```python
from build123d import *

# Parameters (mm, degrees)
SKETCH1_R           = 35
BOSS_EXTRUDE1_DEPTH = 50
SKETCH2_R           = 11.75
CUT_EXTRUDE1_DEPTH  = 21
SKETCH3_R           = 9
CUT_EXTRUDE2_DEPTH  = 5
SKETCH6_R           = 6.35
CUT_EXTRUDE3_DEPTH  = 71.356236397
CUT_EXTRUDE4_START  = -20
SKETCH7_R           = 35
CUT_EXTRUDE4_DEPTH  = 20
SKETCH9_R           = 3.302
CUT_EXTRUDE6_DEPTH  = 58.879184514


with BuildPart() as part:
    # Sketch1 → Boss-Extrude1 (new body)
    with BuildSketch(Plane.XY):
        Circle(SKETCH1_R)
    extrude(amount=BOSS_EXTRUDE1_DEPTH)

    # Sketch2 → Cut-Extrude1 (cut)
    with BuildSketch(Plane.XY.offset(50)):
        with Locations((0, -0.363798412)):
            Circle(SKETCH2_R)
    extrude(amount=-CUT_EXTRUDE1_DEPTH, mode=Mode.SUBTRACT)

    # Sketch3 → Cut-Extrude2 (cut)
    with BuildSketch(Plane.XY.offset(29)):
        Circle(SKETCH3_R)
    extrude(amount=-CUT_EXTRUDE2_DEPTH, mode=Mode.SUBTRACT)

    # Sketch4 → Cut-Revolve1 (revolve, cut)
    with BuildSketch(Plane(origin=(0, 0, 0), x_dir=(0, 0, -1), z_dir=(1, 0, 0))):
        with BuildLine():
            Line((-8.85349547, 5), (-8.85349547, 0))
            Line((-8.85349547, 0), (-29.014540537, 0))
            Line((-29.014540537, 0), (-29.014540537, 8.986487334))
            add(Edge.make_bspline(
                [(-29.014540537, 8.986487334), (-22.084577695, 17.461249934), (-14.611301832, 9.423177176), (-8.85349547, 5)],
                knots=[0, 0, 0, 0, 1, 1, 1, 1], degree=3))
        make_face()
    revolve(axis=Axis((0, 0, 8.85349547), (0, 0, 1)), mode=Mode.SUBTRACT)

    # Sketch6 → Cut-Extrude3 (cut, through all)
    with BuildSketch(Plane(origin=(0, 0, 0), x_dir=(-1, 0, 0), z_dir=(0, 0, -1))):
        Circle(SKETCH6_R)
    extrude(amount=-CUT_EXTRUDE3_DEPTH, mode=Mode.SUBTRACT)

    # Sketch7 → Cut-Extrude4 (cut)
    with BuildSketch(Plane.XY.offset(50).offset(CUT_EXTRUDE4_START)):
        Circle(SKETCH7_R)
    extrude(amount=CUT_EXTRUDE4_DEPTH, mode=Mode.SUBTRACT)

    # Sketch9 → Cut-Extrude6 (cut, through all)
    with BuildSketch(Plane(origin=(0, 0, 0), x_dir=(-1, 0, 0), z_dir=(0, 0, -1))):
        with Locations((0, -23.5)):
            Circle(SKETCH9_R)
        with Locations((-16.617009358, -16.617009358)):
            Circle(SKETCH9_R)
        with Locations((-23.5, 0)):
            Circle(SKETCH9_R)
        with Locations((-16.617009358, 16.617009358)):
            Circle(SKETCH9_R)
        with Locations((0, 23.5)):
            Circle(SKETCH9_R)
        with Locations((16.617009358, 16.617009358)):
            Circle(SKETCH9_R)
        with Locations((23.5, 0)):
            Circle(SKETCH9_R)
        with Locations((16.617009358, -16.617009358)):
            Circle(SKETCH9_R)
    extrude(amount=-CUT_EXTRUDE6_DEPTH, mode=Mode.SUBTRACT)


solid = part.part
```
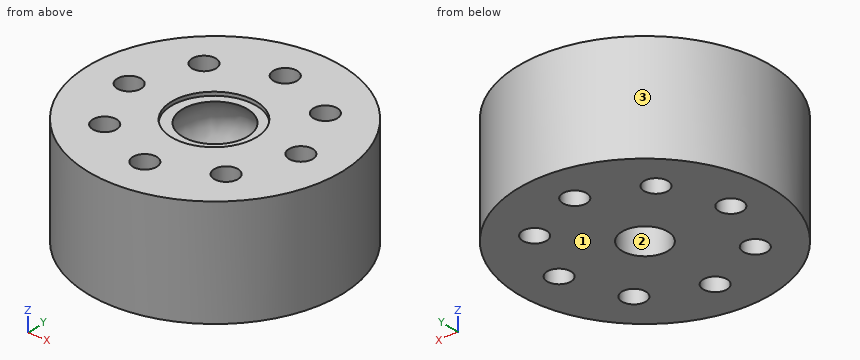
Can you work these out from the model? Positions are in its coordinate system, mm. Face numbers are marked on the shaded views. Round coordinates to 2 decimals unless told otherwise and drop trailing zeros. Loops run counter-clockwise (first coordinate to the right, second up) from the corner with the lowest first, then second, coordinate; pieces in that order, holes last. Notation, with made-up numbers: M -16.75,22 L 35.25,22 A14 ccw 35.25,33 Z; hole C 58.5,-13.5 d3. An arc over 180 degrees is marked long. Answer in a Markdown table with one row per item.
1. If we section it at A-A, the plane y = -23.5: Please give me the cut outline in (x, z), plus the area to 3 significant figures.
Established:
| item | result |
|---|---|
| outline | M -25.94,0 L -3.3,0 L -3.3,30 L -25.94,30 Z; M 3.3,0 L 25.94,0 L 25.94,30 L 3.3,30 Z |
| area | 1,360 mm² |
2. Thinking about a two-plate mould opening in X: for the marked faces 1, 2 and 3, which applies, pulls with the +X half, pulls with the -X half, needs draft (parallel to the pull), parting line crosses it, or undercut?
Established:
| item | result |
|---|---|
| face 1 | needs draft |
| face 2 | undercut |
| face 3 | parting line crosses it |
3. I'm going to push flat-ended pins straight in: pin 1 Ø7.5 at (x, y) = (0, -23.5) entering from -Z; pin 2 Ø8 at (x, z) = (-24.5, 4) entering from -Y; pin 3 Ø4 at (y, z) = (18, 12.5) entering from -X; pin 4 Ø21 at (x, y) = (0, -0.36) entering from +Z. Where does each tip first touch, or does it pass through?
Established:
| item | result |
|---|---|
| pin 1 | z = 0 |
| pin 2 | y = -28.37 |
| pin 3 | x = -31.13 |
| pin 4 | z = 29 |
4. Please list where these lines run through material, in increasing order: line 1 (Y direction, x = -3, z = 12); line 2 (X direction, y = 19, z = 12); line 3 (X direction, y = -18, z = 25). Write a range as from..to.
Established:
| item | result |
|---|---|
| line 1 | -34.87..-24.88, -22.12..-6.91, 6.91..22.12, 24.88..34.87 |
| line 2 | -29.39..-18.9, -14.33..14.33, 18.9..29.39 |
| line 3 | -30.02..-19.62, -13.62..13.62, 19.62..30.02 |
5. If we section it at D-D, the plane y = -15: Please give me the cut outline in (x, z).
Established:
| item | result |
|---|---|
| outline | M -31.62,0 L -19.5,0 L -19.5,30 L -31.62,30 Z; M -13.74,0 L 13.74,0 L 13.74,30 L -13.74,30 Z; M 19.5,0 L 31.62,0 L 31.62,30 L 19.5,30 Z |
6. If we section it at B-B, the plane z = 3.5: Give the number of separate pieces and of enclosed holes in the cut face, plus the area to 3 significant figures.
Established:
| item | result |
|---|---|
| separate pieces | 1 |
| enclosed holes | 9 |
| area | 3,450 mm² |
